For this review, take the finished solid that the model builds, in its own axes (mm). A direction names the side the tool comes from. Round coordinates to 2 decimals unless told otherwise and drop trailing zeros. Write each loop counter-clockwise with the first axis right and the second up, starting at its lowest first coordinate (ties: lowest second). Pieces come first, ordered by that corner, then holes. Notation, with made-up numbers: (43, 82) -> (100, 82) arc R28 cw to (100, 105) -> close; hole circle Ø2 at (87, 28). An arc over 180 degrees is marked (long way). Answer as CSV lines item,"result". Start each with the question number.
Item 1: Mouldability with a two-part tool opening along X and no side actions: class faces 4 (the flat face through (-9.923, -9, 476)), 5 (the flat face through (-12, -11, -12.7)), 6 (the flat face through (-22, 12.874, 476)) as +X half, -X half, draft (parallel to the pull), parting line (faces both ways), or undercut.
Item 2: Take a section at A-A on z = 343. Give the boundary of the cut face in (x, y).
Item 3: Take a section at C-C on z = 800.1. Give the boundary of the cut face in (x, y).
Item 4: Machinability: for faces 1 (the cylindrical face through (-33.758, -8.723, 11.126)), 2 (the flat face through (-13.098, -10, 476)), 3 (the cylindrical face through (-11.49, -14.22, 13.67)), which of the approach directions +Z, -Z, +X, -X, +Y, -Y give a long, thin tool a straight path to every point of the face, cutting with its end or side? Answer none if there is none.
Item 5: Take a section at B-B on z = 25.4. Give the boundary of the cut face in (x, y).
Item 6: Wall thickness on probe 1 along X at (y, z) = (12, 60); probe 2 along Y at (x, z) = (-15.5, 337); probe 3 along Z at (x, y) = (-32.75, -2.5): over which ranges is each line inside the solid? List them lowest first. Write a range as from..to.
Autodesk Inventor part; units mm, degrees
ref_plane "YZ Plane" through (0, 0, 0) normal (1, 0, 0) x (0, 1, 0)
ref_plane "XZ Plane" through (0, 0, 0) normal (0, 1, 0) x (-1, 0, 0)
ref_plane "XY Plane" through (0, 0, 0) normal (0, 0, 1) x (1, 0, 0)
sketch "Sketch1" plane through (0, 0, 0) normal (0, 0, 1) x (1, 0, 0)
  line L0 (-35.3228, 16.049) -> (-9.9228, 16.049)
  line L1 (-9.9228, 16.049) -> (-9.9228, -34.751)
  line L2 (-9.9228, -34.751) -> (-35.3228, -34.751)
  line L3 (-35.3228, -34.751) -> (-35.3228, 16.049)
  line L4 (-13.0978, 12.874) -> (-32.1478, 12.874)
  line L5 (-32.1478, 12.874) -> (-32.1478, -31.576)
  line L6 (-32.1478, -31.576) -> (-13.0978, -31.576)
  line L7 (-13.0978, -31.576) -> (-13.0978, 12.874)
  point P0 (0, 0)
  dimension "d0" = 25.4
  dimension "d1" = 50.8
  dimension "d2" = 3.175
extrude "Extrusion1" add sketch "Sketch1" along normal blind 977.9
sketch "Sketch2" plane through (-35.3228, -34.751, 0) normal (-1, 0, 0) x (0, 0, 1)
  line L0 (0, 0) -> (0, 50.8) construction
  line L1 (0, 25.4) -> (25.4, 25.4) construction
  circle A0 centre (25.4, 25.4) radius 14.2875
  point P0 (0, 34.751)
  dimension "d5" = 25.4
  dimension "d9" = 28.575
extrude "Extrusion2" cut sketch "Sketch2" against normal blind 12.7
sketch "Sketch3" plane through (-35.3228, -34.751, 0) normal (-1, 0, 0) x (0, 0, 1)
  line L0 (977.9, 50.8) -> (977.9, 0) construction
  line L1 (977.9, 25.4) -> (800.1, 25.4) construction
  circle A0 centre (800.1, 25.4) radius 14.2875
  point P0 (0, 34.751)
  dimension "d10" = 177.8
  dimension "d11" = 28.575
extrude "Extrusion3" cut sketch "Sketch3" against normal blind 25.4
sketch "Sketch7" plane through (-9.9228, -34.751, 0) normal (1, 0, 0) x (0, 0, -1)
  line L0 (0, 0) -> (0, 50.8) construction
  line L1 (0, 25.4) -> (-25.4, 25.4) construction
  circle A0 centre (-25.4, 25.4) radius 12.7
  point P0 (0, 34.751)
  dimension "d34" = 25.4
  dimension "d35" = 25.4
extrude "Extrusion7" cut sketch "Sketch7" against normal blind 12.7
sketch "Sketch9" plane through (-9.9228, -34.751, 0) normal (1, 0, 0) x (0, 0, -1)
  circle A0 centre (-25.4, 25.4) radius 12.7 construction
  line L0 (-25.4, 25.4) -> (-25.4, 49.2125) construction
  line L1 (-25.4, 49.2125) -> (-4.7778, 37.3063) construction
  line L2 (-4.7778, 37.3063) -> (-4.7778, 13.4938) construction
  line L3 (-4.7778, 13.4938) -> (-25.4, 1.5875) construction
  line L4 (-25.4, 1.5875) -> (-46.0222, 13.4937) construction
  line L5 (-46.0222, 13.4937) -> (-46.0222, 37.3062) construction
  line L6 (-46.0222, 37.3062) -> (-25.4, 49.2125) construction
  circle A1 centre (-4.7778, 37.3063) radius 2.5797
  circle A2 centre (-4.7778, 13.4938) radius 2.5797
  circle A3 centre (-46.0222, 13.4938) radius 2.5797
  circle A4 centre (-46.0222, 37.3062) radius 2.5797
  point P0 (0, 34.751)
  dimension "d44" = 23.8125
  dimension "d45" = 5.1594
  dimension "d46" = 5.1594
  dimension "d47" = 5.1594
  dimension "d48" = 5.1594
extrude "Extrusion9" cut sketch "Sketch9" against normal blind 25.4
sketch "Sketch10" plane through (0, 0, 0) normal (0, 0, -1) x (-1, 0, 0)
  line L0 (35.3228, 16.049) -> (9.9228, 16.049)
  line L1 (9.9228, 16.049) -> (13.0978, 16.049)
  line L2 (13.0978, 16.049) -> (13.0978, -34.751)
  line L3 (13.0978, -34.751) -> (9.9228, -34.751)
  line L4 (9.9228, -34.751) -> (9.9228, 16.049)
  line L5 (9.9228, -34.751) -> (35.3228, -34.751)
  line L6 (9.9228, -34.751) -> (35.3228, -34.751)
  line L7 (35.3228, -34.751) -> (35.3228, -31.576)
  line L8 (35.3228, -31.576) -> (9.9228, -31.576)
  line L9 (9.9228, -31.576) -> (9.9228, -34.751)
  line L10 (35.3228, -34.751) -> (32.1478, -34.751)
  line L11 (32.1478, -34.751) -> (32.1478, 16.049)
  line L12 (32.1478, 16.049) -> (35.3228, 16.049)
  line L13 (35.3228, 16.049) -> (35.3228, -34.751)
  line L14 (9.9228, 16.049) -> (35.3228, 16.049)
  line L15 (35.3228, 16.049) -> (35.3228, 12.874)
  line L16 (35.3228, 12.874) -> (9.9228, 12.874)
  line L17 (9.9228, 12.874) -> (9.9228, 16.049)
  point P0 (0, 0)
  dimension "d51" = 3.175
  dimension "d52" = 50.8
  dimension "d53" = 25.4
  dimension "d54" = 3.175
  dimension "d55" = 3.175
  dimension "d56" = 50.8
  dimension "d57" = 25.4
  dimension "d58" = 3.175
extrude "Extrusion10" add sketch "Sketch10" along normal blind 12.7 contours L13 L16 L11 L0 | L11 L16 L2 L0 | L13 L8 L11 L16 | L2 L16 L4 L0 | L7 L5 L11 L8 | L2 L8 L4 L16 | L11 L5 L2 L8 | L2 L3 L4 L8
sketch "Sketch11" plane through (-35.3228, 16.049, 977.9) normal (0, 1, 0) x (1, 0, 0)
  line L0 (0, 0) -> (25.4, 0) construction
  line L1 (12.7, 0) -> (12.7, 508) construction
  line L2 (25.4, 0) -> (25.4, 990.6) construction
  line L3 (12.7, 0) -> (520.7, 0) construction
  circle A0 centre (12.7, 508) radius 2.5797
  point P0 (35.3228, 977.9)
  dimension "d61" = 508
  dimension "d62" = 90
  dimension "d63" = 5.1594
extrude "Extrusion11" cut sketch "Sketch11" against normal blind 101.6
properties part number "41.75in Arm Beam Alternate (Left)"
Output values:
1,face 4,"+X half"
1,face 5,"draft"
1,face 6,"undercut"
2,outline,"(-35.32, -34.75) -> (-9.92, -34.75) -> (-9.92, 16.05) -> (-35.32, 16.05) -> close; hole (-32.15, -31.58) -> (-13.1, -31.58) -> (-13.1, 12.87) -> (-32.15, 12.87) -> close"
3,outline,"(-35.32, -34.75) -> (-9.92, -34.75) -> (-9.92, -23.64) -> (-13.1, -23.64) -> (-13.1, -31.58) -> (-32.15, -31.58) -> (-32.15, -23.64) -> (-35.32, -23.64) -> close; (-35.32, 4.94) -> (-32.15, 4.94) -> (-32.15, 12.87) -> (-13.1, 12.87) -> (-13.1, 4.94) -> (-9.92, 4.94) -> (-9.92, 16.05) -> (-35.32, 16.05) -> close"
4,face 1,"-X"
4,face 2,"+Z, -Z"
4,face 3,"+X, -X"
5,outline,"(-35.32, -34.75) -> (-9.92, -34.75) -> (-9.92, -22.05) -> (-13.1, -22.05) -> (-13.1, -31.58) -> (-32.15, -31.58) -> (-32.15, -23.64) -> (-35.32, -23.64) -> close; (-35.32, 4.94) -> (-32.15, 4.94) -> (-32.15, 12.87) -> (-13.1, 12.87) -> (-13.1, 3.35) -> (-9.92, 3.35) -> (-9.92, 16.05) -> (-35.32, 16.05) -> close"
6,probe 1,"x = -35.32..-32.15, -13.1..-9.92"
6,probe 2,"y = -34.75..-31.58, 12.87..16.05"
6,probe 3,"z = -12.7..12.86, 37.94..787.56, 812.64..977.9"
